Here's how the part is built. I have some questions about the finished solid (model axes, mm). A direction names the side the tool comes from. Round coordinates to 2 decimals unless told otherwise and drop trailing zeros. One line per item, written item: value.
```python
from build123d import *

# Parameters (mm, degrees)
SKETCH_1_R          = 2.5
EXTRUDE_1_DEPTH     = 242.72
CUT_EXTRUDE_1_DEPTH = 328.339480429


with BuildPart() as part:
    # 草图1 → 凸台-拉伸1 (new body)
    with BuildSketch(Plane(origin=(0, 0, 0), x_dir=(1, 0, 0), z_dir=(0, 1, 0))):
        with BuildLine():
            Line((-216.919311098, -330.148369359), (-218.719311098, -330.148369359))
            Line((-218.719311098, -330.148369359), (-218.719311098, -335.548369359))
            ThreePointArc((-218.719311098, -335.548369359), (-218.27997127, -336.60902953), (-217.219311098, -337.048369359))
            Line((-217.219311098, -337.048369359), (-211.819311098, -337.048369359))
            Line((-211.819311098, -337.048369359), (-211.819311098, -335.248369359))
            Line((-211.819311098, -335.248369359), (-214.219311098, -335.248369359))
            Line((-214.219311098, -335.248369359), (-214.219311098, -333.445419514))
            Line((-214.219311098, -333.445419514), (-210.922260943, -330.148369359))
            Line((-210.922260943, -330.148369359), (-206.516361253, -330.148369359))
            Line((-206.516361253, -330.148369359), (-203.219311098, -333.445419514))
            Line((-203.219311098, -333.445419514), (-203.219311098, -335.248369359))
            Line((-203.219311098, -335.248369359), (-205.619311098, -335.248369359))
            Line((-205.619311098, -335.248369359), (-205.619311098, -337.048369359))
            Line((-205.619311098, -337.048369359), (-200.219311098, -337.048369359))
            ThreePointArc((-200.219311098, -337.048369359), (-199.158650926, -336.60902953), (-198.719311098, -335.548369359))
            Line((-198.719311098, -335.548369359), (-198.719311098, -330.148369359))
            Line((-198.719311098, -330.148369359), (-200.519311098, -330.148369359))
            Line((-200.519311098, -330.148369359), (-200.519311098, -332.548369359))
            Line((-200.519311098, -332.548369359), (-202.322260943, -332.548369359))
            Line((-202.322260943, -332.548369359), (-205.665184078, -329.205446224))
            Line((-205.665184078, -329.205446224), (-205.665184078, -324.891292493))
            Line((-205.665184078, -324.891292493), (-202.322260943, -321.548369359))
            Line((-202.322260943, -321.548369359), (-200.519311098, -321.548369359))
            Line((-200.519311098, -321.548369359), (-200.519311098, -323.948369359))
            Line((-200.519311098, -323.948369359), (-198.719311098, -323.948369359))
            Line((-198.719311098, -323.948369359), (-198.719311098, -318.548369359))
            ThreePointArc((-198.719311098, -318.548369359), (-199.158650926, -317.487709187), (-200.219311098, -317.048369359))
            Line((-200.219311098, -317.048369359), (-205.619311098, -317.048369359))
            Line((-205.619311098, -317.048369359), (-205.619311098, -318.848369359))
            Line((-205.619311098, -318.848369359), (-203.219311098, -318.848369359))
            Line((-203.219311098, -318.848369359), (-203.219311098, -320.651319203))
            Line((-203.219311098, -320.651319203), (-206.516361253, -323.948369359))
            Line((-206.516361253, -323.948369359), (-210.922260943, -323.948369359))
            Line((-210.922260943, -323.948369359), (-214.219311098, -320.651319203))
            Line((-214.219311098, -320.651319203), (-214.219311098, -318.848369359))
            Line((-214.219311098, -318.848369359), (-211.819311098, -318.848369359))
            Line((-211.819311098, -318.848369359), (-211.819311098, -317.048369359))
            Line((-211.819311098, -317.048369359), (-217.219311098, -317.048369359))
            ThreePointArc((-217.219311098, -317.048369359), (-218.27997127, -317.487709187), (-218.719311098, -318.548369359))
            Line((-218.719311098, -318.548369359), (-218.719311098, -323.948369359))
            Line((-218.719311098, -323.948369359), (-216.919311098, -323.948369359))
            Line((-216.919311098, -323.948369359), (-216.919311098, -321.548369359))
            Line((-216.919311098, -321.548369359), (-215.116361253, -321.548369359))
            Line((-215.116361253, -321.548369359), (-211.773438118, -324.891292493))
            Line((-211.773438118, -324.891292493), (-211.773438118, -329.205446224))
            Line((-211.773438118, -329.205446224), (-215.116361253, -332.548369359))
            Line((-215.116361253, -332.548369359), (-216.919311098, -332.548369359))
            Line((-216.919311098, -332.548369359), (-216.919311098, -330.148369359))
        make_face()
        with Locations(Location((-208.719311098, -327.048369359, 0), (0, 0, 270))):
            Circle(SKETCH_1_R, mode=Mode.SUBTRACT)
    extrude(amount=EXTRUDE_1_DEPTH)

    # 草图2 → 切除-拉伸1 (cut, through all)
    with BuildSketch(Plane.XY.offset(337.048369359)):
        Polygon((-218.719311098, 0), (-198.719311098, 20), (-198.719311098, 0), align=None)
    extrude(amount=-CUT_EXTRUDE_1_DEPTH, mode=Mode.SUBTRACT)


solid = part.part
```
Q1. Which directions (+Z, -Z, +X, -X, +Y, -Y) give clear straight access to the entire face, cutting with the end or side of a thin tool? Please do faces 1 (the face through (-209, 124, 323.948)), 2 (the face through (-211.773, 123, 327)), 3 (the face through (-205.665, 126, 327)).
Answers:
face 1: -Z, +Y, -Y
face 2: -X, +Y, -Y
face 3: +X, +Y, -Y
Q2. If we mould it in two halves opening along Z, with no side actions, what happens to faces 4 (the face through (-207.03, 123.463, 325.206)), 5 (the face through (-203, 126, 337.048)), 6 (the face through (-198.719, 130, 321))? For each: pulls with the +Z half, pulls with the -Z half, needs draft (parallel to the pull), parting line crosses it, or undercut.
Answers:
face 4: undercut
face 5: pulls with the +Z half
face 6: needs draft
Q3. I need wall thicknesses on line 1 along Z through (x, y) = (-216.25, 137.5); line 2 along X through (y, z) = (23.5, 328.25); line 3 along Z through (x, y) = (-203.5, 47). Which ranges of each line are inside material? Lowest first, please.
Answers:
line 1: 317.05 to 321.55, 332.55 to 337.05
line 2: -211.77 to -210.91, -206.53 to -205.67
line 3: 317.05 to 318.85, 320.93 to 322.73, 331.37 to 333.16, 335.25 to 337.05
Q4. For P1, Ø0.9, axis at x = -199, y = 79, coming from the -Z side; P2, Ø3.5, axis at x = -209, y = 146.5, coming from the +Z side; P3, Ø0.5, axis at y = 152, z = 336, coming from the -X side, each with a flat end and sliding along its axis, tell me the tip position at first contact or that it passes through.
Answers:
P1: z = 317.26
P2: z = 330.15
P3: x = -218.71
